```python
from build123d import *

# Parameters (mm, degrees)
SKETCH_1_W          = 235
SKETCH_1_H          = 120
SKETCH_1_R          = 41.65
EXTRUDE_1_DEPTH     = 3
SKETCH_2_R          = 1.65
CUT_EXTRUDE_1_DEPTH = 3
SKETCH_3_R          = 1.5
SKETCH_3_R_2        = 1.65
CUT_EXTRUDE_2_DEPTH = 3
SKETCH_4_R          = 1.5
CUT_EXTRUDE_3_DEPTH = 3
SKETCH_5_R          = 1.5
CUT_EXTRUDE_4_DEPTH = 3
FILLET_1_R          = 2
SKETCH_6_R          = 1.65
CUT_EXTRUDE_5_DEPTH = 10


with BuildPart() as part:
    # 草图1 → 凸台-拉伸1 (new body)
    with BuildSketch(Plane(origin=(0, 0, 0), x_dir=(1, 0, 0), z_dir=(0, 1, 0))):
        Rectangle(SKETCH_1_W, SKETCH_1_H)
        with Locations(Location((-59.15, 0, 0), (0, 0, 270))):
            Circle(SKETCH_1_R, mode=Mode.SUBTRACT)
        with Locations(Location((59.15, 0, 0), (0, 0, 90))):
            Circle(SKETCH_1_R, mode=Mode.SUBTRACT)
    extrude(amount=EXTRUDE_1_DEPTH)

    # 草图2 → 切除-拉伸1 (cut)
    with BuildSketch(Plane(origin=(0, 3, 0), x_dir=(1, 0, 0), z_dir=(0, 1, 0))):
        with Locations(Location((-83.75, -38.869525338, 0), (0, 0, 270))):
            Circle(SKETCH_2_R)
        with Locations(Location((-83.75, 38.869525338, 0), (0, 0, 270))):
            Circle(SKETCH_2_R)
        with Locations(Location((-34.55, 38.869525338, 0), (0, 0, 90))):
            Circle(SKETCH_2_R)
        with Locations(Location((-34.55, -38.869525338, 0), (0, 0, 90))):
            Circle(SKETCH_2_R)
        with Locations(Location((34.55, -38.869525338, 0), (0, 0, 270))):
            Circle(SKETCH_2_R)
        with Locations(Location((83.75, -38.869525338, 0), (0, 0, 90))):
            Circle(SKETCH_2_R)
        with Locations(Location((34.55, 38.869525338, 0), (0, 0, 270))):
            Circle(SKETCH_2_R)
        with Locations(Location((83.75, 38.869525338, 0), (0, 0, 90))):
            Circle(SKETCH_2_R)
    extrude(amount=-CUT_EXTRUDE_1_DEPTH, mode=Mode.SUBTRACT)

    # 草图3 → 切除-拉伸2 (cut)
    with BuildSketch(Plane(origin=(0, 3, 0), x_dir=(1, 0, 0), z_dir=(0, 1, 0))):
        with Locations(Location((-111.5, -28, 0), (0, 0, 270))):
            Circle(SKETCH_3_R)
        with Locations(Location((-111.5, -8, 0), (0, 0, 270))):
            Circle(SKETCH_3_R)
        with Locations(Location((111.5, -8, 0), (0, 0, 90))):
            Circle(SKETCH_3_R)
        with Locations(Location((111.5, -28, 0), (0, 0, 90))):
            Circle(SKETCH_3_R)
        with Locations(Location((-112.5, 55, 0), (0, 0, 270))):
            Circle(SKETCH_3_R)
        with Locations(Location((-92.5, 55, 0), (0, 0, 270))):
            Circle(SKETCH_3_R)
        with Locations(Location((92.5, 55, 0), (0, 0, 90))):
            Circle(SKETCH_3_R)
        with Locations(Location((112.5, 55, 0), (0, 0, 90))):
            Circle(SKETCH_3_R)
        with Locations(Location((103.310016868, -26.5, 0), (0, 0, 270))):
            Circle(SKETCH_3_R_2)
        with Locations(Location((-93.135083269, 50, 0), (0, 0, 270))):
            Circle(SKETCH_3_R_2)
        with Locations(Location((-111, 47.400657923, 0), (0, 0, 270))):
            Circle(SKETCH_3_R_2)
        with Locations(Location((93.135083269, 50, 0), (0, 0, 270))):
            Circle(SKETCH_3_R_2)
        with Locations(Location((111, 47.400657923, 0), (0, 0, 270))):
            Circle(SKETCH_3_R_2)
        with Locations(Location((-95.485573862, -41.374781037, 0), (0, 0, 270))):
            Circle(SKETCH_3_R)
        with Locations(Location((95.485573862, -41.374781037, 0), (0, 0, 270))):
            Circle(SKETCH_3_R)
    extrude(amount=-CUT_EXTRUDE_2_DEPTH, mode=Mode.SUBTRACT)

    # 草图4 → 切除-拉伸3 (cut)
    with BuildSketch(Plane(origin=(0, 3, 0), x_dir=(1, 0, 0), z_dir=(0, 1, 0))):
        with Locations(Location((-112.5, -55, 0), (0, 0, 270))):
            Circle(SKETCH_4_R)
        with Locations(Location((-112.5, 55, 0), (0, 0, 270))):
            Circle(SKETCH_4_R)
        with Locations(Location((112.5, 55, 0), (0, 0, 90))):
            Circle(SKETCH_4_R)
        with Locations(Location((112.5, -55, 0), (0, 0, 270))):
            Circle(SKETCH_4_R)
        with Locations(Location((-34.5, -55, 0), (0, 0, 270))):
            Circle(SKETCH_4_R)
        with Locations(Location((34.5, -55, 0), (0, 0, 270))):
            Circle(SKETCH_4_R)
    extrude(amount=-CUT_EXTRUDE_3_DEPTH, mode=Mode.SUBTRACT)

    # 草图5 → 切除-拉伸4 (cut)
    with BuildSketch(Plane(origin=(0, 3, 0), x_dir=(1, 0, 0), z_dir=(0, 1, 0))):
        with Locations(Location((-8, 55, 0), (0, 0, 270))):
            Circle(SKETCH_5_R)
        with Locations(Location((8, 55, 0), (0, 0, 270))):
            Circle(SKETCH_5_R)
    extrude(amount=-CUT_EXTRUDE_4_DEPTH, mode=Mode.SUBTRACT)

    # 圆角1
    fillet_1_edges = [part.edges().sort_by_distance(p)[0] for p in [
        (117.5, 1.5, 60),
        (-117.5, 1.5, 60),
        (-117.5, 1.5, -60),
        (117.5, 1.5, -60),
    ]]
    fillet(fillet_1_edges, radius=FILLET_1_R)

    # 草图6 → 切除-拉伸5 (cut)
    with BuildSketch(Plane(origin=(0, 3, 0), x_dir=(1, 0, 0), z_dir=(0, 1, 0))):
        with Locations(Location((-103.900657923, -26.5, 0), (0, 0, 270))):
            Circle(SKETCH_6_R)
    extrude(amount=-CUT_EXTRUDE_5_DEPTH, mode=Mode.SUBTRACT)


solid = part.part
```
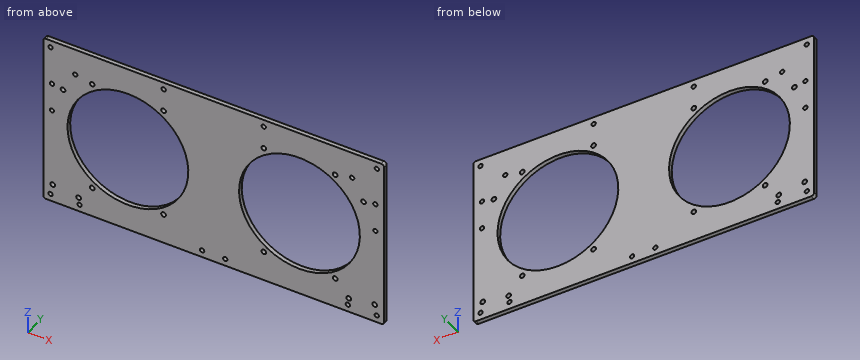
For this review, take the finished solid that the model builds, in its own axes (mm). Coordinates: 2 decimals unless noted, no trailing zeros. Write each loop counter-clockwise with the first axis right and the second up, starting at its lowest first coordinate (ties: lowest second). Pieces come first, ordered by that corner, then holes. Notation, with made-up numbers: (-37, 14.5) - (-25, 14.5) arc R21 cw to (-25, 20.5) - close; hole circle Ø3 at (76, 27.5). An arc over 180 degrees is marked (long way). Put each result on its own line as item: value.
1. Add section A-A, the plane z = 0. Give the boundary of the cut face in (x, y).
Values found:
outline: (-117.5, 0) - (-100.8, 0) - (-100.8, 3) - (-117.5, 3) - close; (-17.5, 0) - (17.5, 0) - (17.5, 3) - (-17.5, 3) - close; (100.8, 0) - (117.5, 0) - (117.5, 3) - (100.8, 3) - close
2. Add section D-D, the plane y = 1.8. Count the separate pieces of the cut face and the enclosed holes in it, then the cut area to 3 significant figures.
Values found:
separate pieces: 1
enclosed holes: 32
area: 17,100 mm²
3. Add section B-B, the plane x = 50. Give the boundary of the cut face in (y, z).
Values found:
outline: (0, -60) - (3, -60) - (3, -40.63) - (0, -40.63) - close; (0, 40.63) - (3, 40.63) - (3, 60) - (0, 60) - close
4. Wall thickness on probe 1 along X at (y, z) = (1.8, -50); probe 2 along X at (y, z) = (0.5, 0); probe 3 along Z at (x, y) = (-92.5, 1.2): over which ranges is each line inside the solid? List them lowest first.
Values found:
probe 1: -117.5 to -94.79, -91.49 to 91.49, 94.79 to 117.5
probe 2: -117.5 to -100.8, -17.5 to 17.5, 100.8 to 117.5
probe 3: -60 to -56.5, -53.5 to -51.52, -48.48 to -24.95, 24.95 to 60
5. Add section C-C, the plane z = 13.5. Give the boundary of the cut face in (x, y), then the cut area to 3 significant figures.
Values found:
outline: (-117.5, 0) - (-98.55, 0) - (-98.55, 3) - (-117.5, 3) - close; (-19.75, 0) - (19.75, 0) - (19.75, 3) - (-19.75, 3) - close; (98.55, 0) - (117.5, 0) - (117.5, 3) - (98.55, 3) - close
area: 232 mm²
6. For pin 1 (2 mm diameter, centred on x = 103.31, z = 26.5, fed in from +Y); pin 2 (4 mm diameter, centred on x = -34.55, z = 38.87, fed in from +Y), all flat-tipped, find the tip position at first contact; note any pin that passes through.
Values found:
pin 1: through
pin 2: y = 3
